Geometry check sheet. Reference: the model listing, model coordinates, mm. A direction names the side the tool comes from. Round coordinates to 2 decimals unless told otherwise and drop trailing zeros. Write each loop counter-clockwise with the first axis right and the second up, starting at its lowest first coordinate (ties: lowest second). Pieces come first, ordered by that corner, then holes. Notation, with made-up numbers: M 24.25,8 L 52.25,8 A11 ccw 52.25,27 Z; hole C 38,12.25 d7. An arc over 180 degrees is marked long. One line per item, written item: value. Start each with the question number.
1. Section check B-B (y = 6.75). Record the boundary of the cut face in (x, z) (3 decimals), and give its area (3 significant figures).
2. Access from +Z, -Z, +X, -X, +Y, -Y to the whole of each face (thin tool, end or side, straight path). Record for faces 5 (the cylindrical face through (6.25, 6.33, -2.87)), 6 (the cylindrical face through (35.87, 6.33, -8.36)), 7 (the flat face through (6, 7.62, -13)), 8 (the cylindrical face through (6.45, 6.33, -22.53)).
3. Section check D-D (y = 2.5). Record the boundary of the cut face in (x, z).
4. Release check for a two-part mould opening along X. For faces 1 (the flat face through (1.905, 6, -13)), 2 (the flat face through (10.795, 6, -13)), 3 (the flat face through (37, 7.62, -13)), 4 (the flat face through (22.8, 2.5, -21.6)) record: pulls with the +X half, pulls with the -X half, needs draft (parallel to the pull), parting line crosses it, or undercut.
5. Depth check by flat-ended pin: P1, Ø12, axis at x = 24, z = -10.5, coming from the +Y side; P2, Ø0.8, axis at y = 6.5, z = -14.5, coming from the -X side (3 decimals); P3, Ø2, axis at y = 6.5, z = -11, coming from the +X side. Enter the tip coordinate at first touch or a pass-through.
6. Section check C-C (x = 6.35). Record the boundary of the cut face in (y, z).
7. Scan lines: probe 1 along Y at (x, z) = (13, -22.75); probe 2 along X at (y, z) = (5.75, -17.5) (3 decimals); probe 3 along X at (y, z) = (5.5, -11.5) (3 decimals). Record each from-to range of solid material in increasing order. Write a range as [from, to].
8. Section check A-A (z = -12.7). Record the boundary of the cut face in (x, y) (3 decimals), and give its area (3 significant figures).
from build123d import *

# Parameters (mm, degrees)
BOSS_EXTRUDE1_DEPTH = 5.08
SKETCH5_R           = 4.445
BOSS_EXTRUDE2_DEPTH = 2.54


with BuildPart() as part:
    # Sketch1 → Boss-Extrude1 (new body)
    with BuildSketch(Plane(origin=(0, 0, 0), x_dir=(1, 0, 0), z_dir=(0, 1, 0))):
        with BuildLine():
            Line((0, 7.495923678), (0, 17.904076322))
            ThreePointArc((0, 17.904076322), (2.24551941, 22.749253211), (7.393933569, 24.167677738))
            Line((7.393933569, 24.167677738), (38.618391502, 18.963601416))
            ThreePointArc((38.618391502, 18.963601416), (43.924457933, 12.7), (38.618391502, 6.436398584))
            Line((38.618391502, 6.436398584), (7.393933569, 1.232322262))
            ThreePointArc((7.393933569, 1.232322262), (2.24551941, 2.650746789), (0, 7.495923678))
        make_face()
    extrude(amount=BOSS_EXTRUDE1_DEPTH)

    # Sketch5 → Boss-Extrude2 (add)
    with BuildSketch(Plane(origin=(0, 5.08, 0), x_dir=(1, 0, 0), z_dir=(0, 1, 0))):
        with BuildLine():
            Line((1.905, 18.086409435), (1.905, 7.313590565))
            ThreePointArc((1.905, 7.313590565), (6.35, 2.868590565), (10.795, 7.313590565))
            Line((10.795, 7.313590565), (10.795, 18.086409435))
            ThreePointArc((10.795, 18.086409435), (6.35, 22.531409435), (1.905, 18.086409435))
        make_face()
        with Locations((36.83, 12.7)):
            Circle(SKETCH5_R)
    extrude(amount=BOSS_EXTRUDE2_DEPTH)


solid = part.part
Result sheet:
1. outline: M 1.905,-18.086 A4.445 ccw 10.795,-18.086 L 10.795,-7.314 A4.445 ccw 1.905,-7.314 Z; C 36.83,-12.7 d8.89
1. area: 220 mm2
2. face 5: +Z, +Y
2. face 6: +Y
2. face 7: +Z, -Z, +X, -X, +Y
2. face 8: -Z, +Y
3. outline: M 0,-17.9 A6.35 ccw 7.39,-24.17 L 38.62,-18.96 A6.35 ccw 38.62,-6.44 L 7.39,-1.23 A6.35 ccw 0,-7.5 Z
4. face 1: pulls with the -X half
4. face 2: undercut
4. face 3: needs draft
4. face 4: pulls with the +X half
5. P1: stops at y = 5.08
5. P2: stops at x = 1.905
5. P3: stops at x = 41.22
6. outline: M 0,-24.25 L 5.08,-24.25 L 5.08,-22.53 L 7.62,-22.53 L 7.62,-2.87 L 5.08,-2.87 L 5.08,-1.15 L 0,-1.15 Z
7. probe 1: y = [0, 5.08]
7. probe 2: x = [1.905, 10.795]
7. probe 3: x = [1.905, 10.795], [32.55, 41.11]
8. outline: M 0,0 L 43.924,0 L 43.924,5.08 L 41.275,5.08 L 41.275,7.62 L 32.385,7.62 L 32.385,5.08 L 10.795,5.08 L 10.795,7.62 L 1.905,7.62 L 1.905,5.08 L 0,5.08 Z
8. area: 268 mm2
